Geometry: final body of the model. Coordinates: model frame, mm. A direction names the side the tool comes from. Give positions to 0.01 mm unless a question says otherwise; leave off trailing zeros. Write each loop counter-clockwise with the first axis right and the second up, starting at its lowest first coordinate (ties: lowest second). Pieces come first, ordered by that corner, then holes.
```python
from build123d import *

# Parameters (mm, degrees)
SKETCH1_R               = 6.35
SKETCH1_R_2             = 3.175
BOSS_EXTRUDE1_DEPTH     = 20
SKETCH2_R               = 10
SKETCH2_R_2             = 3.175
BOSS_EXTRUDE2_DEPTH     = 3.175
SKETCH3_R               = 1.5
CUT_EXTRUDE1_DEPTH      = 10
CUT_EXTRUDE1_DEPTH_BACK = 11
SKETCH4_W               = 6.5
SKETCH4_H               = 0.894727321
CUT_EXTRUDE2_DEPTH      = 13.5


with BuildPart() as part:
    # Sketch1 → Boss-Extrude1 (new body)
    with BuildSketch(Plane(origin=(0, 0, 0), x_dir=(1, 0, 0), z_dir=(0, 1, 0))):
        Circle(SKETCH1_R)
        Circle(SKETCH1_R_2, mode=Mode.SUBTRACT)
    extrude(amount=BOSS_EXTRUDE1_DEPTH)

    # Sketch2 → Boss-Extrude2 (add)
    with BuildSketch(Plane(origin=(0, 20, 0), x_dir=(1, 0, 0), z_dir=(0, 1, 0))):
        Circle(SKETCH2_R)
        Circle(SKETCH2_R_2, mode=Mode.SUBTRACT)
    extrude(amount=BOSS_EXTRUDE2_DEPTH)

    # Sketch3 → Cut-Extrude1 (cut, two sides)
    with BuildSketch(Plane.XY) as cut_extrude1_sk:
        with Locations((0, 10)):
            Circle(SKETCH3_R)
    extrude(amount=CUT_EXTRUDE1_DEPTH, mode=Mode.SUBTRACT)
    extrude(cut_extrude1_sk.sketch, amount=-CUT_EXTRUDE1_DEPTH_BACK, mode=Mode.SUBTRACT)

    # Sketch4 → Cut-Extrude2 (cut)
    with BuildSketch(Plane.XZ):
        with Locations((0, -5.90263634)):
            Rectangle(SKETCH4_W, SKETCH4_H)
        with Locations((0, 5.90263634)):
            Rectangle(SKETCH4_W, SKETCH4_H)
    extrude(amount=-CUT_EXTRUDE2_DEPTH, mode=Mode.SUBTRACT)


solid = part.part
```
Item 1: Section C-C, the plane y = 10. Return the cut outline in (x, z) (3 decimals), plus the area to 3 significant figures.
Found:
outline: (-3.25, -5.455) - (-1.5, -5.455) - (-1.5, -2.798) arc R3.175 cw to (-1.5, 2.798) - (-1.5, 5.455) - (-3.25, 5.455) arc R6.35 ccw to start; (1.5, -5.455) - (3.25, -5.455) arc R6.35 ccw to (3.25, 5.455) - (1.5, 5.455) - (1.5, 2.798) arc R3.175 cw to (1.5, -2.798) - close
area: 72.7 mm2
Item 2: Line query: L1, parallel to Y at x = 0, z = -3.9 (3 decimals); L2, parallel to X at y = 7, z = 0 (3 decimals); L3, parallel to Y at x = 4, z = -7.25 (3 decimals). Output: solid intervals per line, ascending.
Found:
L1: y = 0 to 8.5, 11.5 to 23.175
L2: x = -6.35 to -3.175, 3.175 to 6.35
L3: y = 20 to 23.175
Item 3: Reachability of faces 1 (the face through (1.5, 11.4, 2.8)), 2 (the face through (0, 13.5, -6)), 3 (the face through (0, 7, 5.455)), 4 (the face through (-4.68, 9.86, -4.29)) from +Z, -Z, +X, -X, +Y, -Y: full face, straight path, thin tool, end or side. Return the list, or none.
Found:
face 1: +Y, -Y
face 2: -Z, +X, -X, -Y
face 3: +Z, +X, -X, -Y
face 4: -Y
Item 4: Pin query (flat end, axial travel): pin 1 Ø7 at (x, y) = (0, 9) entering from -Z; pin 2 Ø5 at (x, y) = (0, 5) entering from +Z; pin 3 Ø5.5 at (x, z) = (0, 0) entering from -Y; pin 4 Ø12 at (x, y) = (0, 10) entering from +Z. Return the tip coordinate at first contact, or that it passes through.
Found:
pin 1: stops at z = -5.46
pin 2: stops at z = 5.46
pin 3: passes through
pin 4: stops at z = 6.35
Item 5: Section A-A, the plane x = 0. Return the cut outline in (y, z) (3 decimals).
Found:
outline: (0, -5.455) - (8.5, -5.455) - (8.5, -3.175) - (0, -3.175) - close; (0, 3.175) - (8.5, 3.175) - (8.5, 5.455) - (0, 5.455) - close; (11.5, -5.455) - (13.5, -5.455) - (13.5, -6.35) - (20, -6.35) - (20, -10) - (23.175, -10) - (23.175, -3.175) - (11.5, -3.175) - close; (11.5, 3.175) - (23.175, 3.175) - (23.175, 10) - (20, 10) - (20, 6.35) - (13.5, 6.35) - (13.5, 5.455) - (11.5, 5.455) - close
Item 6: Section D-D, the plane y = 4.25. Return the cut outline in (x, z) (3 decimals).
Found:
outline: (-3.25, -5.455) - (3.25, -5.455) arc R6.35 ccw to (3.25, 5.455) - (-3.25, 5.455) arc R6.35 ccw to start; hole circle Ø6.35 at (0, 0)
Item 7: Pull-direction query (Y, two-part tool) for faces 5 (the face through (0, 13.5, 6)), 6 (the face through (0, 7, -5.455)), 7 (the face through (1.386, 9.425, 4.108)); classes: +Y half, -Y half, draft (parallel to the pull), parting line (faces both ways), or undercut.
Found:
face 5: -Y half
face 6: draft
face 7: undercut
Item 8: Section B-B, the plane z = 0. Return the cut outline in (x, y) (3 decimals).
Found:
outline: (-10, 20) - (-6.35, 20) - (-6.35, 0) - (-3.175, 0) - (-3.175, 23.175) - (-10, 23.175) - close; (3.175, 0) - (6.35, 0) - (6.35, 20) - (10, 20) - (10, 23.175) - (3.175, 23.175) - close
